The figure shows three views and two pictorial views of one solid part (mm, origin at its lowest corner). Answer the questions. A direction names the side the tool comes from. Coordinates: 2 decimals unless noted, no trailing zeros. Loops run counter-clockwise (first coordinate to the right, second up) from the corner with the lowest first, then second, coordinate; pieces in that order, holes last. Notation, with made-up numbers: (-18, -35.75) -> (-9, -35.75) arc R14 cw to (-9, -12.75) -> close; hole circle Ø6 at (46, 34.25). An arc over 180 degrees is marked (long way). Answer in a Markdown table with one row per item.
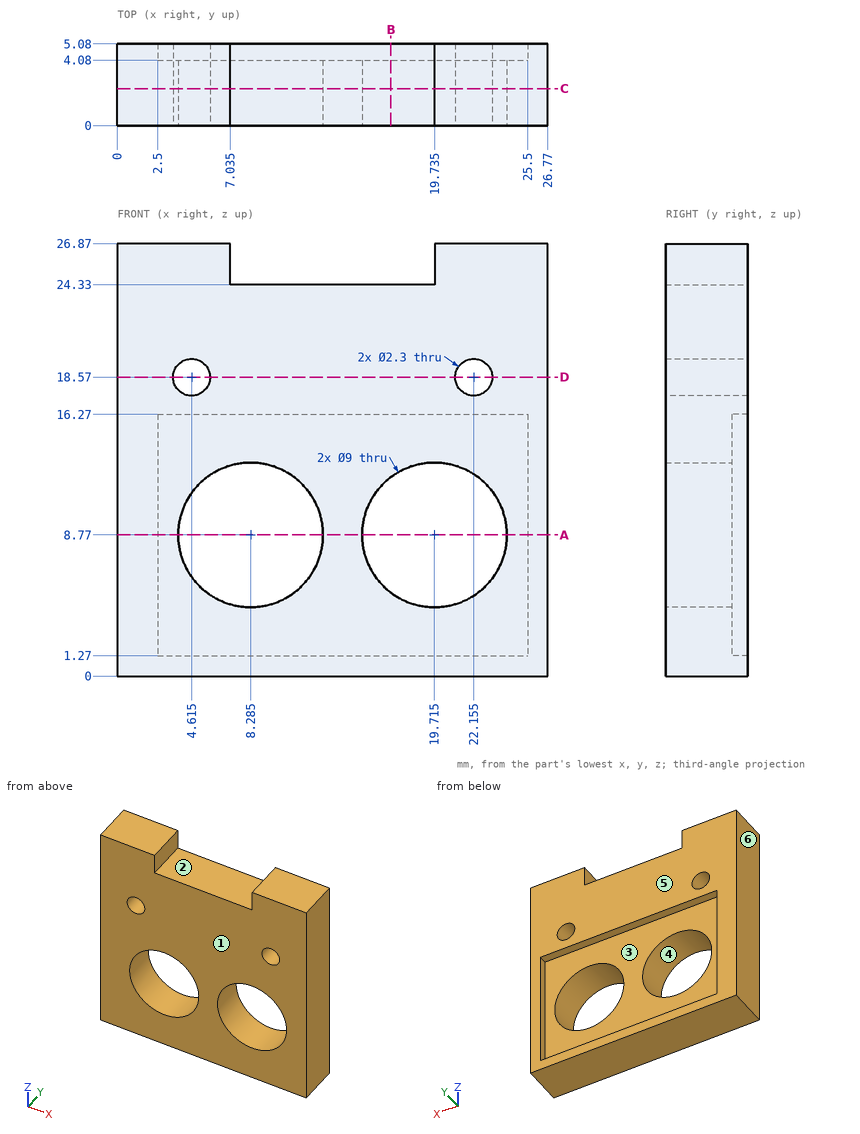
Item 1: A cutting plane is placed at D-D, the plane z = 18.57. Determine the outline of the cut face in (x, y) (3 decimals).
Findings below:
| item | result |
|---|---|
| outline | (0, 0) -> (3.465, 0) -> (3.465, 5.08) -> (0, 5.08) -> close; (5.765, 0) -> (21.005, 0) -> (21.005, 5.08) -> (5.765, 5.08) -> close; (23.305, 0) -> (26.77, 0) -> (26.77, 5.08) -> (23.305, 5.08) -> close |
Item 2: Find the intervals of material crossed by probe 1 along X at (y, z) = (2.4, 18.57) (3 decimals); probe 2 along X at (y, z) = (2, 8.77) (3 decimals); probe 3 along Z at (x, y) = (7.25, 4.4), in increasing order.
Findings below:
| item | result |
|---|---|
| probe 1 | x = 0 to 3.465, 5.765 to 21.005, 23.305 to 26.77 |
| probe 2 | x = 0 to 3.785, 12.785 to 15.215, 24.215 to 26.77 |
| probe 3 | z = 0 to 1.27, 16.27 to 24.33 |
Item 3: A cutting plane is placed at C-C, the plane y = 2.3. Determine the outline of the cut face in (x, z) (3 decimals), plus the area to 3 significant figures.
Findings below:
| item | result |
|---|---|
| outline | (0, 0) -> (26.77, 0) -> (26.77, 26.87) -> (19.735, 26.87) -> (19.735, 24.33) -> (7.035, 24.33) -> (7.035, 26.87) -> (0, 26.87) -> close; hole circle Ø2.3 at (4.615, 18.57); hole circle Ø9 at (8.285, 8.77); hole circle Ø9 at (19.715, 8.77); hole circle Ø2.3 at (22.155, 18.57) |
| area | 552 mm2 |
Item 4: A cutting plane is placed at B-B, the plane x = 17. Determine the outline of the cut face in (y, z), plus the area to 3 significant figures.
Findings below:
| item | result |
|---|---|
| outline | (0, 0) -> (5.08, 0) -> (5.08, 1.27) -> (4.08, 1.27) -> (4.08, 5.18) -> (0, 5.18) -> close; (0, 12.36) -> (4.08, 12.36) -> (4.08, 16.27) -> (5.08, 16.27) -> (5.08, 24.33) -> (0, 24.33) -> close |
| area | 79.3 mm2 |
Item 5: Determine the mould class of the marked faces 4, 5 and 6 for opening direction X: +X half, -X half, draft (parallel to the pull), parting line (faces both ways), or undercut.
Findings below:
| item | result |
|---|---|
| face 4 | undercut |
| face 5 | draft |
| face 6 | -X half |
Item 6: A tool of negligible diameter and unlimited length cuts with its end or side. For the marked faces 1, 2 and 3, from which of +Z, -Z, +X, -X, +Y, -Y can it reach the whole face along a straight path? Write none if from no direction.
Findings below:
| item | result |
|---|---|
| face 1 | +Z, -Z, +X, -X, -Y |
| face 2 | +Z, +Y, -Y |
| face 3 | +Y |
Item 7: A flat-ended cylindrical pin translates along its axis: pin 1 Ø2 at (x, y) = (10.5, 1) entering from +Z. Find the tip coordinate at first contact, or state that the pin passes through.
Findings below:
| item | result |
|---|---|
| pin 1 | stops at z = 24.33 |
Item 8: A cutting plane is placed at A-A, the plane z = 8.77. Determine the outline of the cut face in (x, y) (3 decimals), plus the area to 3 significant figures.
Findings below:
| item | result |
|---|---|
| outline | (0, 0) -> (3.785, 0) -> (3.785, 4.08) -> (2.5, 4.08) -> (2.5, 5.08) -> (0, 5.08) -> close; (12.785, 0) -> (15.215, 0) -> (15.215, 4.08) -> (12.785, 4.08) -> close; (24.215, 0) -> (26.77, 0) -> (26.77, 5.08) -> (25.5, 5.08) -> (25.5, 4.08) -> (24.215, 4.08) -> close |
| area | 39.6 mm2 |
